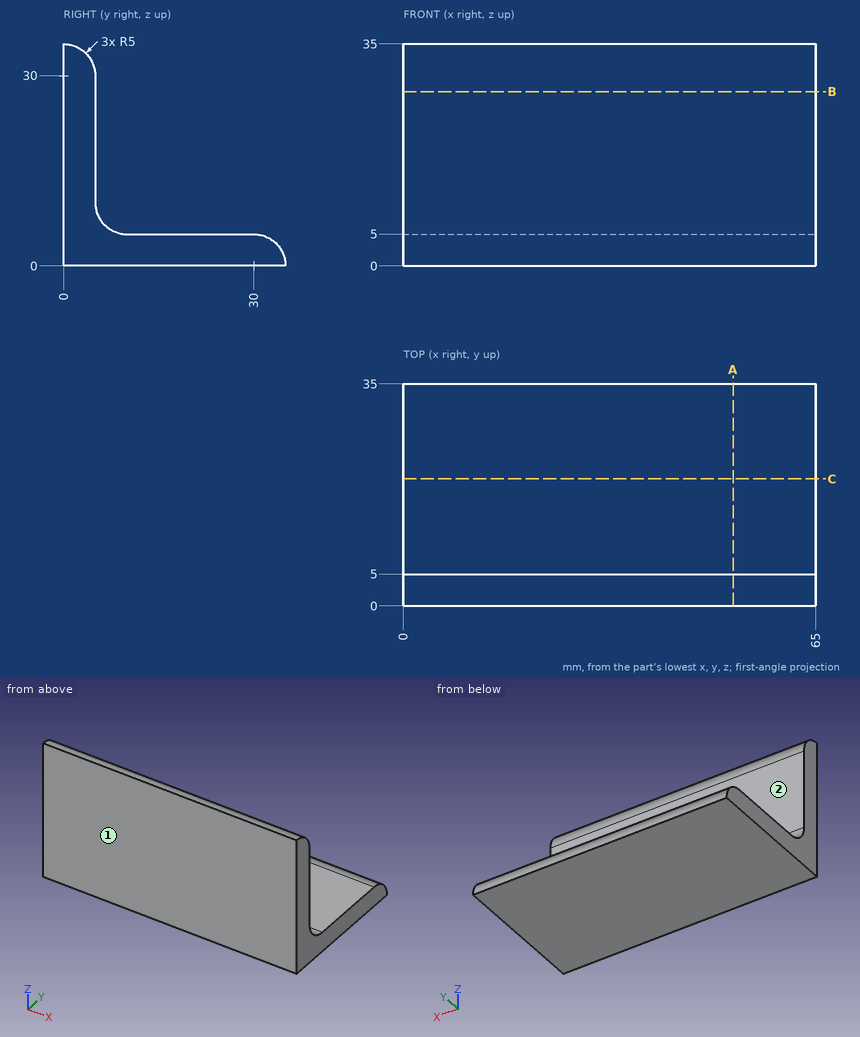
Geometry check sheet. Reference: drawing and pictorial views, mm from the part's lowest x, y, z. A direction names the side the tool comes from. Round coordinates to 2 decimals unless told otherwise and drop trailing zeros. Loops run counter-clockwise (first coordinate to the right, second up) from the corner with the lowest first, then second, coordinate; pieces in that order, holes last. Notation, with made-up numbers: (60.25, -26) -> (102.25, -26) arc R21 cw to (102.25, -13) -> close; hole circle Ø4 at (-23, -33.75). An arc over 180 degrees is marked (long way). Answer as a JSON object with one key per item and string values.
Q1. Section check B-B (z = 27.5). Record the boundary of the cut face in (x, y).
Data:
{"outline": "(0, 0) -> (65, 0) -> (65, 5) -> (0, 5) -> close"}
Q2. Section check A-A (x = 52). Record the boundary of the cut face in (y, z), then the cut area to 3 significant figures.
Data:
{"outline": "(0, 0) -> (35, 0) arc R5 ccw to (30, 5) -> (10, 5) arc R5 cw to (5, 10) -> (5, 30) arc R5 ccw to (0, 35) -> close", "area": "320 mm2"}
Q3. Scan lines: line 1 (Z direction, x = 60, y = 24.5); line 2 (Y direction, x = 36, z = 32.5). Record each from-to range of solid material in increasing order. Write a range as from..to.
Data:
{"line 1": "z = 0..5", "line 2": "y = 0..4.33"}
Q4. Access from +Z, -Z, +X, -X, +Y, -Y to the whole of each face (thin tool, end or side, straight path). Record for the marked faces 1 and 2.
Data:
{"face 1": "+Z, -Z, +X, -X, -Y", "face 2": "+Z, +X, -X, +Y"}
Q5. Go/stop test with flat-tipped pins: P1, Ø12, axis at x = 8, z = 31, coming from the -Y side; P2, Ø10, axis at y = 25, z = 11.5, coming from the +X side; P3, Ø10, axis at x = 45, y = 20.5, coming from the +Z side; P4, Ø1.5, axis at x = 41.5, z = 9, coming from the +Y side. Record where each tip stops, or that it passes through.
Data:
{"P1": "stops at y = 0", "P2": "passes through", "P3": "stops at z = 5", "P4": "stops at y = 5.32"}
